Input: part model. Units: mm. Frame: model coordinates. Face numbers are marked on the shaded views. A direction names the side the tool comes from. Coordinates: 2 decimals unless noted, no trailing zeros. Write each loop counter-clockwise with the first axis right and the second up, starting at its lowest first coordinate (ties: lowest second). Pieces come first, ordered by that corner, then holes. Notation, with made-up numbers: (49, -23) -> (56, -23) arc R23 cw to (56, 16) -> close; hole circle Ø10 at (84.25, -26). An arc over 180 degrees is marked (long way). One line per question, with ' | ' between items. Start each with the question number.
```python
from build123d import *

# Parameters (mm, degrees)
SKETCH_W        = 108
SKETCH_H        = 75.2
SKETCH_W_2      = 91
SKETCH_H_2      = 57
PAD_DEPTH       = 2
PAD001_DEPTH    = 14
POCKET_DEPTH    = 75.2
POCKET001_DEPTH = 108
SKETCH004_W     = 8.5
SKETCH004_H     = 9.1
PAD002_DEPTH    = 14
SKETCH005_R     = 1.55
POCKET002_DEPTH = 30
FILLET_R        = 1
FILLET001_R     = 1
FILLET002_R     = 1
FILLET003_R     = 1


with BuildPart() as part:
    # Sketch → Pad (new body)
    with BuildSketch(Plane.XY):
        Rectangle(SKETCH_W, SKETCH_H)
        Rectangle(SKETCH_W_2, SKETCH_H_2, mode=Mode.SUBTRACT)
    extrude(amount=PAD_DEPTH)

    # Sketch001 (on Face10 of Pad) → Pad001 (join)
    with BuildSketch(Plane.XY.offset(2)):
        Polygon((-54, 37.6), (-54, 14.5), (-45.5, 14.5), (-45.5, 28.5), (-31.5, 28.5), (-31.5, 37.6), align=None)
        Polygon((31.5, 37.6), (54, 37.6), (54, 14.5), (45.5, 14.5), (45.5, 28.5), (31.5, 28.5), align=None)
        Polygon((45.5, -14.5), (45.5, -28.5), (31.5, -28.5), (31.5, -37.6), (54, -37.6), (54, -14.5), align=None)
        Polygon((-31.5, -28.5), (-45.5, -28.5), (-45.5, -14.5), (-54, -14.5), (-54, -37.6), (-31.5, -37.6), align=None)
    extrude(amount=PAD001_DEPTH)

    # Sketch002 (on Face25 of Pad001) → Pocket (cut)
    with BuildSketch(Plane.XZ.offset(37.6)):
        Polygon((-45.5, 16), (-31.5, 16), (-31.5, 2), align=None)
        Polygon((31.5, 16), (31.5, 2), (45.5, 16), align=None)
    extrude(amount=-POCKET_DEPTH, mode=Mode.SUBTRACT)

    # Sketch003 (on Face14 of Pocket) → Pocket001 (cut)
    with BuildSketch(Plane.YZ.offset(54)):
        Polygon((-28.5, 16), (-14.5, 16), (-14.5, 2), align=None)
        Polygon((14.5, 2), (14.5, 16), (28.5, 16), align=None)
    extrude(amount=-POCKET001_DEPTH, mode=Mode.SUBTRACT)

    # Sketch004 (on Face26 of Pocket001) → Pad002 (join)
    with BuildSketch(Plane.XY.offset(16)):
        with Locations((-49.75, 33.05)):
            Rectangle(SKETCH004_W, SKETCH004_H)
        with Locations((49.75, 33.05)):
            Rectangle(SKETCH004_W, SKETCH004_H)
        with Locations((49.75, -33.05)):
            Rectangle(SKETCH004_W, SKETCH004_H)
        with Locations((-49.75, -33.05)):
            Rectangle(SKETCH004_W, SKETCH004_H)
    extrude(amount=PAD002_DEPTH)

    # Sketch005 (on Face51 of Pad002) → Pocket002 (cut)
    with BuildSketch(Plane.XY.offset(30)):
        with Locations((-49.75, 33.05)):
            Circle(SKETCH005_R)
        with Locations((49.75, 33.05)):
            Circle(SKETCH005_R)
        with Locations((49.75, -33.05)):
            Circle(SKETCH005_R)
        with Locations((-49.75, -33.05)):
            Circle(SKETCH005_R)
    extrude(amount=-POCKET002_DEPTH, mode=Mode.SUBTRACT)

    # Fillet
    fillet_edges = [part.edges().sort_by_distance(p)[0] for p in [
        (-54, -37.6, 23),
    ]]
    fillet(fillet_edges, radius=FILLET_R)

    # Fillet001
    fillet001_edges = [part.edges().sort_by_distance(p)[0] for p in [
        (54, -37.6, 23),
    ]]
    fillet(fillet001_edges, radius=FILLET001_R)

    # Fillet002
    fillet002_edges = [part.edges().sort_by_distance(p)[0] for p in [
        (54, 37.6, 9),
    ]]
    fillet(fillet002_edges, radius=FILLET002_R)

    # Fillet003
    fillet003_edges = [part.edges().sort_by_distance(p)[0] for p in [
        (-54, 37.6, 23),
    ]]
    fillet(fillet003_edges, radius=FILLET003_R)


solid = part.part
```
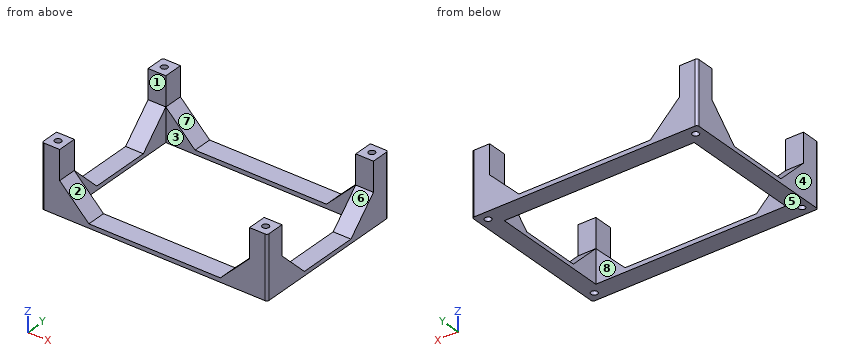
1) Access query for the marked faces 5, 6, 7 and 8. Directions: +Z, -Z, +X, -X, +Y, -Y. A direction counts if a zero-diameter tool reaches every point of the face in a straight line with its end or side. Return the directions, or none.
2) Ray query, line 1 (Y direction, x = -49.75, z = 23.75); line 2 (X direction, y = -34, z = 12.25); line 3 (Y direction, x = 49.75, z = 11.25). Return the intervals inside material, ascending.
3) Section C-C, the plane y = 33.05. Return loops of the section in (x, z), then the cut area to 3 significant figures.
4) Section B-B, the plane y = -16. Return loops of the section in (x, z), then the cut area to 3 significant figures.
5) First-contact query: P1, Ø7.5, axis at x = 8, y = 31.5, coming from the +Z side. Flat tip, straight axial feed; report the tip coordinate or a pass-through.
6) Section A-A, the plane z = 5.25. Give the number of separate pieces and of enclosed holes in the cut face, then the cut area to 3 significant figures.
7) Section D-D, the plane x = -49.75. Return loops of the section in (y, z).
8) Pull-direction query (X, two-part tool) for the marked faces 1, 2, 3 and 4; classes: released by +X, released by -X, zero draft, split by the parting line, or undercut.
Answer block:
1) face 5: -Z, +X, -X, +Y, -Y | face 6: +Z, +X, -X | face 7: +Z, +Y, -Y | face 8: +Z, -Z
2) line 1: y = -37.6 to -34.6, -31.5 to -28.5, 28.5 to 31.5, 34.6 to 37.6 | line 2: x = -54 to -50.97, -48.53 to -41.75, 41.75 to 48.53, 50.97 to 54 | line 3: y = -37.6 to -34.6, -31.5 to -23.75, 23.75 to 31.5, 34.6 to 37.6
3) outline: (-54, 0) -> (-51.3, 0) -> (-51.3, 30) -> (-54, 30) -> close; (-48.2, 0) -> (48.2, 0) -> (48.2, 30) -> (45.5, 30) -> (45.5, 16) -> (31.5, 2) -> (-31.5, 2) -> (-45.5, 16) -> (-45.5, 30) -> (-48.2, 30) -> close; (51.3, 0) -> (54, 0) -> (54, 30) -> (51.3, 30) -> close | area: 702 mm2
4) outline: (-54, 0) -> (-45.5, 0) -> (-45.5, 3.5) -> (-54, 3.5) -> close; (45.5, 0) -> (54, 0) -> (54, 3.5) -> (45.5, 3.5) -> close | area: 59.5 mm2
5) P1: stops at z = 2
6) separate pieces: 4 | enclosed holes: 4 | area: 1,040 mm2
7) outline: (-37.6, 0) -> (-34.6, 0) -> (-34.6, 30) -> (-37.6, 30) -> close; (-31.5, 0) -> (31.5, 0) -> (31.5, 30) -> (28.5, 30) -> (28.5, 16) -> (14.5, 2) -> (-14.5, 2) -> (-28.5, 16) -> (-28.5, 30) -> (-31.5, 30) -> close; (34.6, 0) -> (37.6, 0) -> (37.6, 30) -> (34.6, 30) -> close
8) face 1: zero draft | face 2: undercut | face 3: undercut | face 4: released by -X
